Source: CAD feature listing. Evaluate the final solid. Frame: model axes, mm. Round coordinates to 2 decimals unless told otherwise and drop trailing zeros. Loops run counter-clockwise (first coordinate to the right, second up) from the corner with the lowest first, then second, coordinate; pieces in that order, holes last. Notation, with made-up numbers: (-6.75, 77) - (14.25, 77) arc R20 cw to (14.25, 85) - close; hole circle Ø9 at (-32.75, 14). An arc over 180 degrees is marked (long way). One line per question, with ' | ' between items. Start each with the question number.
1. Cut plane B-B (z = 1.5). State how many separate pieces and enclosed holes the cut face has, then the cut area to 3 significant figures.
2. Cut plane C-C (x = 5.2). Return loops of the section in (y, z).
3. Mould query, pull axis Y, two halves, no side actions, for faces 1 (the cylindrical face through (157.01, 15.23, 1.52)), 2 (the flat face through (114, 20, 3)). Classes: pulls with the +Y half, pulls with the -Y half, needs draft (parallel to the pull), parting line crosses it, or undercut.
4. Cut plane A-A (x = 155.4). Return loops of the section in (y, z), then the cut area to 3 significant figures.
5. Ray query, line 1 (Y direction, x = 170.2, z = 1.7); line 2 (Y direction, x = 130, z = 2.1). Return the intervals inside material, ascending.
```python
from build123d import *

# Parameters (mm, degrees)
F0_W     = 230.4
F0_H     = 40
F1_DEPTH = 3
F2_R     = 2
F3_DEPTH = 3.001
F4_R     = 3
F5_DEPTH = 3.001


with BuildPart() as f1:
    # F0 (on Top) → F1 (new body)
    with BuildSketch(Plane.XY):
        with Locations((115.2, 20)):
            Rectangle(F0_W, F0_H)
    extrude(amount=F1_DEPTH)

    # F2 (on face) → F3 (cut, through all)
    with BuildSketch(Plane.XY.offset(3)):
        with Locations((5.2, 28)):
            Circle(F2_R)
        with Locations((60.2, 28)):
            Circle(F2_R)
        with Locations((115.2, 28)):
            Circle(F2_R)
        with Locations((170.2, 28)):
            Circle(F2_R)
        with Locations((225.2, 28)):
            Circle(F2_R)
    extrude(amount=-F3_DEPTH, mode=Mode.SUBTRACT)

    # F4 (on face) → F5 (cut, through all)
    with BuildSketch(Plane.XY.offset(3)):
        with Locations((20, 12.7)):
            Circle(F4_R)
        with Locations((45.4, 12.7)):
            Circle(F4_R)
        with Locations((75, 12.7)):
            Circle(F4_R)
        with Locations((100.4, 12.7)):
            Circle(F4_R)
        with Locations((130, 12.7)):
            Circle(F4_R)
        with Locations((155.4, 12.7)):
            Circle(F4_R)
        with Locations((185, 12.7)):
            Circle(F4_R)
        with Locations((210.4, 12.7)):
            Circle(F4_R)
    extrude(amount=-F5_DEPTH, mode=Mode.SUBTRACT)


solid = f1.part
```
Answers follow:
1) separate pieces: 1 | enclosed holes: 13 | area: 8,930 mm2
2) outline: (0, 0) - (26, 0) - (26, 3) - (0, 3) - close; (30, 0) - (40, 0) - (40, 3) - (30, 3) - close
3) face 1: undercut | face 2: needs draft
4) outline: (0, 0) - (9.7, 0) - (9.7, 3) - (0, 3) - close; (15.7, 0) - (40, 0) - (40, 3) - (15.7, 3) - close | area: 102 mm2
5) line 1: y = 0 to 26, 30 to 40 | line 2: y = 0 to 9.7, 15.7 to 40
